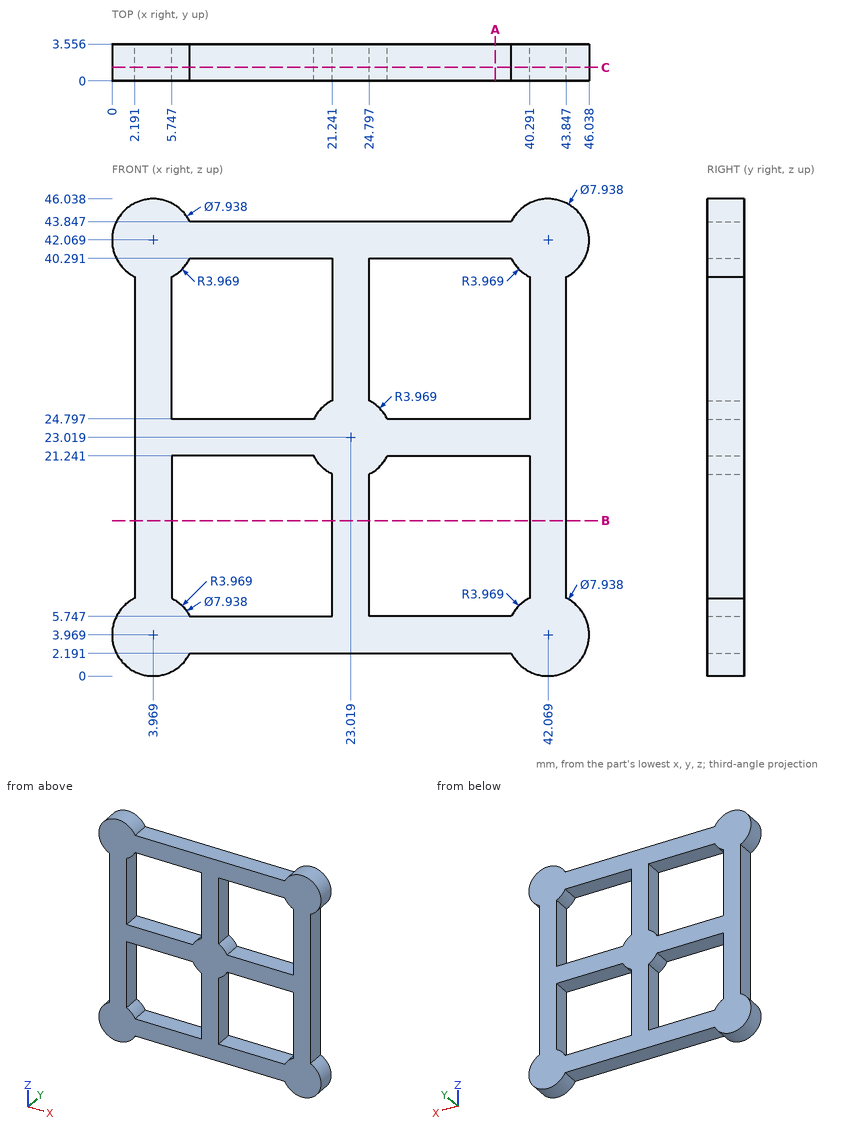
Study the drawing (mm; zero at the part's minimum x, y, z) and answer. Coordinates: 2 decimals unless noted, no trailing zeros. Loops run counter-clockwise (first coordinate to the right, second up) from the corner with the lowest first, then second, coordinate; pieces in that order, holes last. Notation, with made-up numbers: M 86,-32 L 107,-32 A19 cw 107,-20 Z; hole C 21,62.25 d3. An arc over 180 degrees is marked long. Answer as a JSON object with one key per item and string values. Group by question number.
Item 1: Consider L1, parallel to Z at x = 28.5, y = 2.1; L2, parallel to Z at x = 21, y = 1.65 (1 decimal). Determine where each line is inside the solid, lowest interval first.
Item 2: Section B-B (z = 15) is taken. Write down the section's boundary in (x, y) (1 decimal).
Item 3: Section C-C (y = 1.3) is taken. Give the number of separate pieces and of enclosed holes in the cut face.
Item 4: Section A-A (x = 37) is taken. Write down the section's boundary in (y, z) (1 decimal).
Item 5: Each of these flat-tipped pins is pushed along its axis until it touches: P1, Ø1.8, axis at x = 14, y = 1.5, coming from the +Z side; P2, Ø1.5, axis at x = 40, z = 25.5, coming from the -Y side; P3, Ø1.1, axis at y = 1, z = 12.5, coming from the -X side; P4, Ø1.1, axis at y = 1, z = 32.5, coming from the +X side. Where does it stop, or does it pass through?
Solved:
{
 "1": {"L1": "z = 2.19 to 5.75, 21.24 to 24.8, 40.29 to 43.85", "L2": "z = 2.2 to 5.7, 19.6 to 26.4, 40.3 to 43.8"},
 "2": {"outline": "M 2.2,0 L 5.7,0 L 5.7,3.6 L 2.2,3.6 Z; M 21.2,0 L 24.8,0 L 24.8,3.6 L 21.2,3.6 Z; M 40.3,0 L 43.8,0 L 43.8,3.6 L 40.3,3.6 Z"},
 "3": {"separate pieces": "1", "enclosed holes": "4"},
 "4": {"outline": "M 0,2.2 L 3.6,2.2 L 3.6,5.7 L 0,5.7 Z; M 0,21.2 L 3.6,21.2 L 3.6,24.8 L 0,24.8 Z; M 0,40.3 L 3.6,40.3 L 3.6,43.8 L 0,43.8 Z"},
 "5": {"P1": "stops at z = 43.85", "P2": "stops at y = 0", "P3": "stops at x = 2.19", "P4": "stops at x = 43.85"}
}
